```python
from build123d import *

# Parameters (mm, degrees)
BOSS_EXTRUDE1_DEPTH = 6
BOSS_EXTRUDE2_START = 1.7
BOSS_EXTRUDE2_DEPTH = 1.7
CUT_EXTRUDE3_DEPTH  = 29
BOSS_EXTRUDE5_DEPTH = 1.7
CUT_EXTRUDE4_DEPTH  = 85.274737764
SKETCH17_R          = 1.45
BOSS_EXTRUDE6_DEPTH = 2


with BuildPart() as part:
    # Sketch1 → Boss-Extrude1 (new body)
    with BuildSketch(Plane.XY):
        with BuildLine():
            Line((-65.499084074, 50.331718091), (-14.793168506, 50.331718091))
            Line((-14.793168506, 50.331718091), (-5.047168405, 50.331718091))
            ThreePointArc((-5.047168405, 50.331718091), (-2.58785102, 49.313035476), (-1.569168405, 46.853718091))
            Line((-1.569168405, 46.853718091), (-1.569168405, 43.965718386))
            Line((-1.569168405, 43.965718386), (-1.569168405, 33.805718061))
            Line((-1.569168405, 33.805718061), (-1.569168405, 30.881718108))
            ThreePointArc((-1.569168405, 30.881718108), (-2.58785102, 28.422400723), (-5.047168405, 27.403718108))
            Line((-5.047168405, 27.403718108), (-14.829168757, 27.403718108))
            Line((-14.829168757, 27.403718108), (-65.499083667, 27.403718108))
            ThreePointArc((-65.499083667, 27.403718108), (-67.778855129, 28.348030366), (-68.723167387, 30.627801828))
            Line((-68.723167387, 30.627801828), (-68.723167387, 47.107634778))
            ThreePointArc((-68.723167387, 47.107634778), (-67.778855248, 49.387405952), (-65.499084074, 50.331718091))
        make_face()
        with BuildLine():
            Line((-3.269168405, 43.965718386), (-3.269168405, 46.853718091))
            ThreePointArc((-3.269168405, 46.853718091), (-3.789932548, 48.110953948), (-5.047168405, 48.631718091))
            Line((-5.047168405, 48.631718091), (-14.793168506, 48.631718091))
            Line((-14.793168506, 48.631718091), (-65.499084074, 48.631718091))
            ThreePointArc((-65.499084074, 48.631718091), (-66.57677372, 48.185324424), (-67.023167387, 47.107634778))
            Line((-67.023167387, 47.107634778), (-67.023167387, 30.627801828))
            ThreePointArc((-67.023167387, 30.627801828), (-66.576773601, 29.550111894), (-65.499083667, 29.103718108))
            Line((-65.499083667, 29.103718108), (-14.829168757, 29.103718108))
            Line((-14.829168757, 29.103718108), (-5.047168405, 29.103718108))
            ThreePointArc((-5.047168405, 29.103718108), (-3.789932548, 29.624482251), (-3.269168405, 30.881718108))
            Line((-3.269168405, 30.881718108), (-3.269168405, 33.805718061))
            Line((-3.269168405, 33.805718061), (-3.269168405, 43.965718386))
        make_face(mode=Mode.SUBTRACT)
    extrude(amount=-BOSS_EXTRUDE1_DEPTH)

    # Sketch3 → Boss-Extrude2 (add)
    with BuildSketch(Plane.XY.offset(BOSS_EXTRUDE2_START)):
        with BuildLine():
            Line((-68.723167387, 47.107634778), (-68.723167387, 30.627801828))
            ThreePointArc((-68.723167387, 30.627801828), (-67.778855129, 28.348030366), (-65.499083667, 27.403718108))
            Line((-65.499083667, 27.403718108), (-5.047168405, 27.403718108))
            ThreePointArc((-5.047168405, 27.403718108), (-2.58785102, 28.422400723), (-1.569168405, 30.881718108))
            Line((-1.569168405, 30.881718108), (-1.569168405, 46.853718091))
            ThreePointArc((-1.569168405, 46.853718091), (-2.58785102, 49.313035476), (-5.047168405, 50.331718091))
            Line((-5.047168405, 50.331718091), (-65.499084074, 50.331718091))
            ThreePointArc((-65.499084074, 50.331718091), (-67.778855248, 49.387405952), (-68.723167387, 47.107634778))
        make_face()
    extrude(amount=-BOSS_EXTRUDE2_DEPTH)

    # Sketch11 → Cut-Extrude3 (cut)
    with BuildSketch(Plane(origin=(0, 50.331718091, 0), x_dir=(1, 0, 0), z_dir=(0, 1, 0))):
        Polygon((-35.27312624, 6), (-33.77312624, 4.5), (-6.547168405, 4.5), (-5.047168405, 3), (-5.047168405, 0), (-1.569168405, 0), (-1.569168405, 6), align=None)
    extrude(amount=-CUT_EXTRUDE3_DEPTH, mode=Mode.SUBTRACT)

    # Sketch13 → Revolve3 (revolve)
    with BuildSketch(Plane(origin=(0, 0, -2.25), x_dir=(-1, 0, 0), z_dir=(0, 0, -1))):
        with BuildLine():
            Line((8.547168405, 29.103718108), (8.547168405, 30.103718108))
            ThreePointArc((8.547168405, 30.103718108), (9.254275186, 29.810824889), (9.547168405, 29.103718108))
            Line((9.547168405, 29.103718108), (8.547168405, 29.103718108))
        make_face()
    revolve3 = revolve(axis=Axis((-8.547168405, 29.103718108, -2.25), (0, 1, 0)))

    # Mirror3: Revolve3 across plane
    add(revolve3.mirror(Plane(origin=(0, 38.867718099, 0), x_dir=(0, 0, 1), z_dir=(0, -1, 0))))

    # Sketch14 → Boss-Extrude5 (add)
    with BuildSketch(Plane(origin=(0, 0, -6), x_dir=(-1, 0, 0), z_dir=(0, 0, -1))):
        with BuildLine():
            Line((63.723167387, 27.403718108), (63.723167387, 50.331718091))
            Line((63.723167387, 50.331718091), (65.499084074, 50.331718091))
            ThreePointArc((65.499084074, 50.331718091), (67.778855248, 49.387405952), (68.723167387, 47.107634778))
            Line((68.723167387, 47.107634778), (68.723167387, 30.627801828))
            ThreePointArc((68.723167387, 30.627801828), (67.778855129, 28.348030366), (65.499083667, 27.403718108))
            Line((65.499083667, 27.403718108), (63.723167387, 27.403718108))
        make_face()
    extrude(amount=BOSS_EXTRUDE5_DEPTH)

    # Sketch15 → Cut-Extrude4 (cut, through all)
    with BuildSketch(Plane.ZY.offset(68.723167387)):
        with BuildLine():
            ThreePointArc((-2.341753072, 42.182977625), (-3.416753072, 41.107977625), (-2.341753072, 40.032977625))
            Line((-2.341753072, 40.032977625), (-2.341753072, 42.182977625))
        make_face()
        with BuildLine():
            Line((-2.341753072, 42.182977625), (-2.341753072, 40.032977625))
            ThreePointArc((-2.341753072, 40.032977625), (-1.581613282, 40.347837835), (-1.266753072, 41.107977625))
            ThreePointArc((-1.266753072, 41.107977625), (-1.581613282, 41.868117415), (-2.341753072, 42.182977625))
        make_face()
        with BuildLine():
            ThreePointArc((-2.341753072, 37.718380266), (-3.416753072, 36.643380266), (-2.341753072, 35.568380266))
            Line((-2.341753072, 35.568380266), (-2.341753072, 37.718380266))
        make_face()
        with BuildLine():
            Line((-2.341753072, 37.718380266), (-2.341753072, 35.568380266))
            ThreePointArc((-2.341753072, 35.568380266), (-1.581613282, 35.883240476), (-1.266753072, 36.643380266))
            ThreePointArc((-1.266753072, 36.643380266), (-1.581613282, 37.403520056), (-2.341753072, 37.718380266))
        make_face()
    extrude(amount=-CUT_EXTRUDE4_DEPTH, mode=Mode.SUBTRACT)

    # Sketch17 → Boss-Extrude6 (add)
    with BuildSketch(Plane(origin=(0, 0, 0), x_dir=(-1, 0, 0), z_dir=(0, 0, -1))):
        with Locations(Location((14.904168421, 32.641718081, 0), (0, 0, 180))):
            Circle(SKETCH17_R)
        with Locations(Location((60.982168421, 45.218718081, 0), (0, 0, 180))):
            Circle(SKETCH17_R)
    extrude(amount=BOSS_EXTRUDE6_DEPTH)


solid = part.part
```
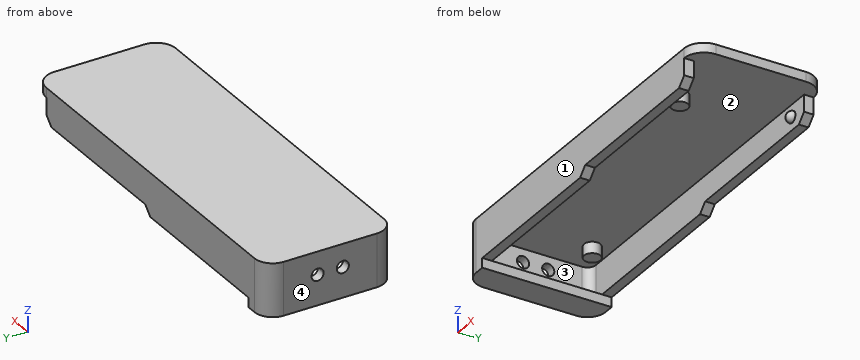
Design review of the part built by this model. Coordinates are the model's own, in mm. Face numbers are marked on the shaded views. Give positions to 0.01 mm unless a question says otherwise; leave off trailing zeros. Order: outer loops, then holes, each group sorted by start corner. A loop starts at its lowest first (then second) coordinate and runs counter-clockwise, first axis right, second up. Notation, with made-up numbers: M -32.5,7 L 10.5,7 A17 cw 10.5,40 Z; hole C 69.5,88.25 d6. An arc over 180 degrees is marked long. One line per question, with ' | ' between items. Start each with the question number.
Q1. We need section C-C (z = -6.75). Write out the cut boundary in (x, y), plus the area to 3 significant figures.
Q2. We need section B-B (y = 44.5). Write out the cut boundary in (x, z).
Q3. For L1, parallel to Z at x = -66, y = 41.75; L2, parallel to Y at x = -58.5, z = -3.5; L3, parallel to Z at x = -15, y = 34, list the stretches that pass through material, from the lowest coordinate up. Write a range as [from, to].
Q4. For pin 1 Ø0.5 at (y, z) = (28, -2) entering from +X; pin 2 Ø0.8 at (x, y) = (-55.5, 50) entering from -Z; pin 3 Ø1.9 at (x, y) = (-20.5, 28) entering from -Z, all flat-tipped, find the tip position at first contact; note any pin that passes through.
Q5. The part is to be moulded in two halves that separate along Y. For the marked faces 1, 2, 3 and 4, say which applies: +Y half, -Y half, draft (parallel to the pull), parting line (faces both ways), or undercut.
Q6. We need section D-D (y = 33.5). Write out the cut boundary in (x, z), plus the area to 3 significant figures.
Q7. We need section A-A (x = -12.5). Write out the cut boundary in (y, z), plus the area to 3 significant figures.
Returned:
1) outline: M -68.72,30.63 A3.22 ccw -65.5,27.4 L -63.72,27.4 L -63.72,50.33 L -65.5,50.33 A3.22 ccw -68.72,47.11 Z | area: 110 mm2
2) outline: M -68.72,-7.7 L -63.72,-7.7 L -63.72,-6 L -67.02,-6 L -67.02,0 L -62.24,0 L -62.24,-2 L -59.72,-2 L -59.72,0 L -1.57,0 L -1.57,1.7 L -68.72,1.7 Z
3) L1: [-7.7, -6], [0, 1.7] | L2: [27.4, 29.1], [48.63, 50.33] | L3: [-2, 1.7]
4) pin 1: x = -5.05 | pin 2: z = -6 | pin 3: z = -4.5
5) face 1: -Y half | face 2: undercut | face 3: undercut | face 4: draft
6) outline: M -68.72,-7.7 L -63.72,-7.7 L -63.72,-6 L -67.02,-6 L -67.02,0 L -16.07,0 L -16.07,-2 L -13.74,-2 L -13.74,0 L -1.57,0 L -1.57,1.7 L -68.72,1.7 Z | area: 138 mm2
7) outline: M 27.4,-4.5 L 29.1,-4.5 L 29.1,0 L 48.63,0 L 48.63,-4.5 L 50.33,-4.5 L 50.33,1.7 L 27.4,1.7 Z | area: 54.3 mm2
